Autodesk Inventor part; units mm, degrees
ref_plane "YZ Plane" through (0, 0, 0) normal (1, 0, 0) x (0, 1, 0)
ref_plane "XZ Plane" through (0, 0, 0) normal (0, 1, 0) x (-1, 0, 0)
ref_plane "XY Plane" through (0, 0, 0) normal (0, 0, 1) x (1, 0, 0)
sketch "main" plane through (0, 0, 0) normal (0, 0, 1) x (1, 0, 0)
  circle A0 centre (-11.3817, -22.2219) radius 2.0955
  circle A1 centre (-11.3817, 28.5781) radius 2.0955
  circle A2 centre (-24.0817, 28.5781) radius 2.0955
  arc A3 (-24.0817, 34.9281) -> (-24.0817, 22.2281) centre (-24.0817, 28.5781) ccw
  line L0 (-4.5584, -27.8865) -> (31.9434, 24.9697)
  line L1 (26.7183, 34.9281) -> (-24.0817, 34.9281)
  arc A4 (31.9434, 24.9697) -> (26.7183, 34.9281) centre (26.7183, 28.5781) ccw
  circle A5 centre (26.7183, 28.5781) radius 2.0955
  arc A6 (-5.8647, -28.5719) -> (-4.5584, -27.8865) centre (-5.8647, -26.9844) ccw
  line L2 (-36.7817, -15.8719) -> (-36.7817, -15.8719)
  line L3 (-36.7817, -28.5719) -> (-5.8647, -28.5719)
  circle A7 centre (-36.7817, -22.2219) radius 2.0955
  arc A8 (-36.7817, -15.8719) -> (-36.7817, -28.5719) centre (-36.7817, -22.2219) ccw
  line L4 (-17.7317, 15.8781) -> (-17.7317, -3.1719)
  line L5 (-30.4317, -15.8719) -> (-36.7817, -15.8719)
  line L6 (-24.0817, 22.2281) -> (-24.0817, 22.2281)
  arc A9 (-17.7317, 15.8781) -> (-24.0817, 22.2281) centre (-24.0817, 15.8781) ccw
  arc A10 (-30.4317, -15.8719) -> (-17.7317, -3.1719) centre (-30.4317, -3.1719) ccw
  circle A11 centre (1.3183, -5.2886) radius 2.0955
  circle A12 centre (14.0183, 11.6448) radius 2.0955
  point P0 (-15.5195, 2.5641)
  point P1 (-17.7317, 22.2281)
  dimension "d0" = 4.191
  dimension "d1" = 4.191
  dimension "d4" = 1.5875
  dimension "d7" = 6.35
  dimension "d8" = 12.7
  dimension "d11" = 4.191
  dimension "d13" = 4.191
sketch "Sketch1" plane through (0, 0, 0) normal (0, 0, 1) x (1, 0, 0)
  circle A0 centre (25.4, 0) radius 2.0955
  circle A1 centre (25.4, 50.8) radius 2.0955
  circle A2 centre (12.7, 50.8) radius 2.0955
  arc A3 (12.7, 57.15) -> (12.7, 44.45) centre (12.7, 50.8) ccw
  line L0 (32.2233, -5.6646) -> (68.7251, 47.1916)
  line L1 (63.5, 57.15) -> (12.7, 57.15)
  arc A4 (68.7251, 47.1916) -> (63.5, 57.15) centre (63.5, 50.8) ccw
  circle A5 centre (63.5, 50.8) radius 2.0955
  arc A6 (30.917, -6.35) -> (32.2233, -5.6646) centre (30.917, -4.7625) ccw
  line L2 (0, 6.35) -> (0, 6.35)
  line L3 (0, -6.35) -> (30.917, -6.35)
  circle A7 centre (0, 0) radius 2.0955
  arc A8 (0, 6.35) -> (0, -6.35) centre (0, 0) ccw
  line L4 (19.05, 38.1) -> (19.05, 19.05)
  line L5 (6.35, 6.35) -> (0, 6.35)
  line L6 (12.7, 44.45) -> (12.7, 44.45)
  arc A9 (19.05, 38.1) -> (12.7, 44.45) centre (12.7, 38.1) ccw
  arc A10 (6.35, 6.35) -> (19.05, 19.05) centre (6.35, 19.05) ccw
  circle A11 centre (38.1, 16.9333) radius 2.0955
  circle A12 centre (50.8, 33.8667) radius 2.0955
extrude "Extrusion1" add sketch "Sketch1" along normal blind 1.5875
equation "\"BendRadius\" = Thickness"
equation "\"BendReliefWidth\" = Thickness"
equation "\"BendReliefDepth\" = 0.5 * Thickness"
equation "\"CornerReliefSize\" = 4 * Thickness"
equation "\"MinimumRemnant\" = 2 * Thickness"
equation "\"TransitionRadius\" = BendRadius"
equation "\"JacobiRadiusSize\" = BendRadius"
equation "\"GapSize\" = Thickness"
properties part number "gusset" material "Acetal Resin, White"
Can you work these out from the model? Positions are in its coordinate system, mm. A direction names the side the tool comes from. Coordinates: 2 decimals unless noted, no trailing zeros. Write each loop counter-clockwise with the first axis right and the second up, starting at its lowest first coordinate (ties: lowest second). Pieces come first, ordered by that corner, then holes. Notation, with made-up numbers: (42.25, 2.25) -> (47.25, 2.25) arc R19 ccw to (47.25, 39.25) -> close; hole circle Ø7 at (66, 52.25). An arc over 180 degrees is marked (long way). Answer as CSV lines item,"result".
1) On a 3-axis mill with a long thin cutter (end or side, diameter ignored), from which of +Z, -Z, +X, -X, +Y, -Y can I reach the whole of each face in a straight line? I mean faces 4 (the flat face through (19.05, 29, 1)), 5 (the flat face through (31, 26, 0)). Say none if no direction works.
Check result:
face 4,"+Z, -Z, -X"
face 5,"-Z, +X, -X, +Y, -Y"
2) If we mould it in two halves opening along X, with no side actions, what happens to faces 1 (the cylindrical face through (63.046, 52.846, 0.783)), 2 (the flat face through (3, 6.35, 1)), 3 (the cylindrical face through (-6.35, -0.14, 0.78))? For each: +X half, -X half, draft (parallel to the pull), parting line (faces both ways), or undercut.
Check result:
face 1,"undercut"
face 2,"draft"
face 3,"-X half"
3) If we section it at C-C on z = 1: Please give me the cut outline in (x, y).
Check result:
outline,"(0, -6.35) -> (30.92, -6.35) arc R1.59 ccw to (32.22, -5.66) -> (68.73, 47.19) arc R6.35 ccw to (63.5, 57.15) -> (12.7, 57.15) arc R6.35 ccw to (12.7, 44.45) arc R6.35 cw to (19.05, 38.1) -> (19.05, 19.05) arc R12.7 cw to (6.35, 6.35) -> (0, 6.35) arc R6.35 ccw to start; hole circle Ø4.19 at (0, 0); hole circle Ø4.19 at (12.7, 50.8); hole circle Ø4.19 at (25.4, 0); hole circle Ø4.19 at (25.4, 50.8); hole circle Ø4.19 at (38.1, 16.93); hole circle Ø4.19 at (50.8, 33.87); hole circle Ø4.19 at (63.5, 50.8)"
4) If I drill on line 1 (Y direction, x = 25.4, z = 0.9); line 2 (X direction, y = 52.5, z = 0.75); line 3 (X direction, y = 1.5, z = 1), over which ranges is the centre line in solid material (lowest first)? Write a range as from..to.
Check result:
line 1,"-6.35..-2.1, 2.1..48.7, 52.9..57.15"
line 2,"6.58..11.47, 13.93..24.17, 26.63..62.27, 64.73..69.62"
line 3,"-6.17..-1.46, 1.46..23.94, 26.86..37.17"
5) Will these pins go through, and if not, where does the flat tip stop? P1, Ø0.5, axis at y = 24, z = 1, coming from the -X side; P2, Ø4, axis at x = 63.5, y = 50.8, coming from the -Z side.
Check result:
P1,"x = 19.05"
P2,"through"
6) If we section it at B-B on x = 26.5: Please give me the cut outline in (y, z), then the cut area to 3 significant figures.
Check result:
outline,"(-6.35, 0) -> (-1.78, 0) -> (-1.78, 1.59) -> (-6.35, 1.59) -> close; (1.78, 0) -> (49.02, 0) -> (49.02, 1.59) -> (1.78, 1.59) -> close; (52.58, 0) -> (57.15, 0) -> (57.15, 1.59) -> (52.58, 1.59) -> close"
area,"89.5 mm²"
7) If we section it at A-A on x = 50.8: Please give me the cut outline in (y, z), then the cut area to 3 significant figures.
Check result:
outline,"(21.24, 0) -> (31.77, 0) -> (31.77, 1.59) -> (21.24, 1.59) -> close; (35.96, 0) -> (57.15, 0) -> (57.15, 1.59) -> (35.96, 1.59) -> close"
area,"50.4 mm²"
8) If we section it at D-D on y = 23.5: Please give me the cut outline in (x, z), then the cut area to 3 significant figures.
Check result:
outline,"(19.05, 0) -> (52.36, 0) -> (52.36, 1.59) -> (19.05, 1.59) -> close"
area,"52.9 mm²"
